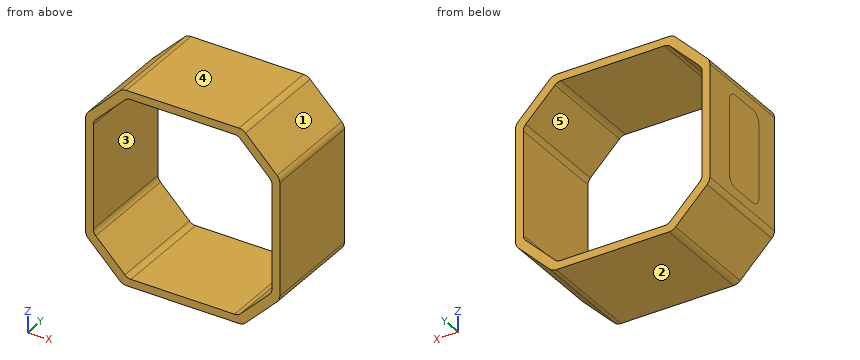
Autodesk Inventor part; units mm, degrees
ref_plane "YZ Plane" through (0, 0, 0) normal (1, 0, 0) x (0, 1, 0)
ref_plane "XZ Plane" through (0, 0, 0) normal (0, 1, 0) x (-1, 0, 0)
ref_plane "XY Plane" through (0, 0, 0) normal (0, 0, 1) x (1, 0, 0)
sketch "Sketch1" plane through (0, 0, 0) normal (0, 1, 0) x (-1, 0, 0)
  line L0 (21, -21) -> (-21, -21)
  line L1 (-21, -21) -> (-21, 21)
  line L2 (-21, 21) -> (21, 21)
  line L3 (21, 21) -> (21, -21)
  line L4 (21, -21) -> (-21, 21) construction
  line L5 (-21, -21) -> (21, 21) construction
  point P0 (0, 0)
  dimension "d0" = 42
  dimension "d1" = 42
extrude "Extrusion1" add sketch "Sketch1" along normal blind 22
chamfer "Chamfer1" distance 8 angle 45 4 edges at (21, 11, 21) (-21, 11, 21) (-21, 11, -21) (21, 11, -21)
fillet "Fillet1" radius 2 8 edges at (-13, 11, -21) (-21, 11, -13) (-21, 11, 13) (-13, 11, 21) (13, 11, 21) (21, 11, 13) (13, 11, -21) (21, 11, -13)
sketch "Sketch4" plane through (0, 22, 0) normal (0, 1, 0) x (1, 0, 0)
  arc A0 (21, 12.1716) -> (20.4142, 13.5858) centre (19, 12.1716) ccw
  line L0 (13.5858, 20.4142) -> (20.4142, 13.5858)
  arc A1 (13.5858, 20.4142) -> (12.1716, 21) centre (12.1716, 19) ccw
  line L1 (12.1716, 21) -> (-12.1716, 21)
  arc A2 (-12.1716, 21) -> (-13.5858, 20.4142) centre (-12.1716, 19) ccw
  line L2 (-20.4142, 13.5858) -> (-13.5858, 20.4142)
  arc A3 (-20.4142, 13.5858) -> (-21, 12.1716) centre (-19, 12.1716) ccw
  line L3 (-21, 12.1716) -> (-21, -12.1716)
  arc A4 (-21, -12.1716) -> (-20.4142, -13.5858) centre (-19, -12.1716) ccw
  line L4 (-13.5858, -20.4142) -> (-20.4142, -13.5858)
  arc A5 (-13.5858, -20.4142) -> (-12.1716, -21) centre (-12.1716, -19) ccw
  line L5 (-12.1716, -21) -> (12.1716, -21)
  arc A6 (12.1716, -21) -> (13.5858, -20.4142) centre (12.1716, -19) ccw
  line L6 (20.4142, -13.5858) -> (13.5858, -20.4142)
  arc A7 (20.4142, -13.5858) -> (21, -12.1716) centre (19, -12.1716) ccw
  line L7 (21, -12.1716) -> (21, 12.1716)
  arc A8 (19.32, 11.1978) -> (18.7811, 12.4989) centre (17.48, 11.1978) ccw
  line L8 (12.4989, 18.7811) -> (18.7811, 12.4989)
  arc A9 (12.4989, 18.7811) -> (11.1978, 19.32) centre (11.1978, 17.48) ccw
  line L9 (11.1978, 19.32) -> (-11.1978, 19.32)
  arc A10 (-11.1978, 19.32) -> (-12.4989, 18.7811) centre (-11.1978, 17.48) ccw
  line L10 (-18.7811, 12.4989) -> (-12.4989, 18.7811)
  arc A11 (-18.7811, 12.4989) -> (-19.32, 11.1978) centre (-17.48, 11.1978) ccw
  line L11 (-19.32, 11.1978) -> (-19.32, -11.1978)
  arc A12 (-19.32, -11.1978) -> (-18.7811, -12.4989) centre (-17.48, -11.1978) ccw
  line L12 (-12.4989, -18.7811) -> (-18.7811, -12.4989)
  arc A13 (-12.4989, -18.7811) -> (-11.1978, -19.32) centre (-11.1978, -17.48) ccw
  line L13 (-11.1978, -19.32) -> (11.1978, -19.32)
  arc A14 (11.1978, -19.32) -> (12.4989, -18.7811) centre (11.1978, -17.48) ccw
  line L14 (18.7811, -12.4989) -> (12.4989, -18.7811)
  arc A15 (18.7811, -12.4989) -> (19.32, -11.1978) centre (17.48, -11.1978) ccw
  line L15 (19.32, -11.1978) -> (19.32, 11.1978)
  point P0 (0, 0)
  point P1 (0, 0)
extrude "Extrusion2" cut sketch "Sketch4" against normal up to surface (22 mm away) contours L15 A15 L14 A14 L13 A13 L12 A12 L11 A11 L10 A10 L9 A9 L8 A8
sketch "Sketch5" plane through (-21, 0, -12.1716) normal (-1, 0, 0) x (0, 0, 1)
  line L0 (2.1716, 15.3239) -> (22.1716, 15.3239)
  line L1 (22.1716, 15.3239) -> (22.1716, 5.3239)
  line L2 (22.1716, 5.3239) -> (2.1716, 5.3239)
  line L3 (2.1716, 5.3239) -> (2.1716, 15.3239)
  line L4 (2.1716, 15.3239) -> (22.1716, 5.3239) construction
  line L5 (22.1716, 15.3239) -> (2.1716, 5.3239) construction
  point P0 (12.1716, 0)
  point P1 (12.1716, 10.3239)
  dimension "d18" = 20
  dimension "d19" = 10
  dimension "d20" = 10
extrude "Extrusion3" add sketch "Sketch5" along normal blind 0.001
sketch "Sketch6" plane through (-21.001, 0, -12.1716) normal (-1, 0, 0) x (0, 0, 1)
  line L0 (2.7184, 14.6945) -> (21.7293, 14.6945) construction
  line L1 (21.7293, 14.6945) -> (21.7293, 6.3236) construction
  line L2 (21.7293, 6.3236) -> (2.7184, 6.3236) construction
  line L3 (2.7184, 6.3236) -> (2.7184, 14.6945) construction
  point P0 (12.1716, 0)
fillet "Fillet2" radius 2 4 edges at (-21.0005, 15.3239, -10) (-21.0005, 5.3239, -10) (-21.0005, 5.3239, 10) (-21.0005, 15.3239, 10)
Could you check a few things on this model? Use its own coordinates, in mm. Face numbers are marked on the shaded views. A direction names the side the tool comes from. Give positions to 0.01 mm unless a question says otherwise; leave off trailing zeros. Loops run counter-clockwise (first coordinate to the right, second up) from the corner with the lowest first, then second, coordinate; pieces in that order, holes last. Notation, with made-up numbers: (25.5, -2) -> (36.5, -2) arc R21 ccw to (36.5, 13) -> close; hole circle Ø7 at (-25, 32). An arc over 180 degrees is marked (long way). Put each result on its own line as item: value.
(1) Imagine slicing it at B-B on x = 4.5. Write out the boundary of the cut face in (y, z), plus the area to 3 significant figures.
Computed:
outline: (0, -21) -> (22, -21) -> (22, -19.32) -> (0, -19.32) -> close; (0, 19.32) -> (22, 19.32) -> (22, 21) -> (0, 21) -> close
area: 73.9 mm^2
(2) For the marked faces 4 and 5, which set-ups out of +Z, -Z, +X, -X, +Y, -Y let a thin tool reach every point of the face, with its end or its side?
Computed:
face 4: +Z, +X, -X, +Y, -Y
face 5: +Y, -Y
(3) I'm going to push a flat-ended pin straight in: pin 1 Ø4 at (x, z) = (-15, 13) entering from +Y. Where does the tip first touch, or does it pass through?
Computed:
pin 1: through
(4) Imagine slicing it at A-A on z = 15. Write out the boundary of the cut face in (x, y), plus the area to 3 significant figures.
Computed:
outline: (-19, 0) -> (-16.28, 0) -> (-16.28, 22) -> (-19, 22) -> close; (16.28, 0) -> (19, 0) -> (19, 22) -> (16.28, 22) -> close
area: 120 mm^2
(5) Please list where these lines run through material, in increasing order: probe 1 along Z at (x, y) = (-10, 4.5); probe 2 along Z at (x, y) = (-14.5, 13). Write a range as [from, to].
Computed:
probe 1: [-21, -19.32], [19.32, 21]
probe 2: [-19.5, -16.78], [16.78, 19.5]
(6) Thinking about a two-plate mould opening in X: for the marked faces 1, 2 and 3, which applies, pulls with the +X half, pulls with the -X half, needs draft (parallel to the pull), parting line crosses it, or undercut?
Computed:
face 1: pulls with the +X half
face 2: needs draft
face 3: undercut
